The model under review builds one solid part; all positions refer to its coordinate system, in mm. Coordinates: 2 decimals unless noted, no trailing zeros. Order: outer loops, then holes, each group sorted by start corner. A loop starts at its lowest first (then second) coordinate and runs counter-clockwise, first axis right, second up. Notation, with made-up numbers: M 36,56 L 88,56 A20 ccw 88,79 Z; hole C 61,14.25 d4. An arc over 180 degrees is marked long. Answer in a Markdown table with one row per item.
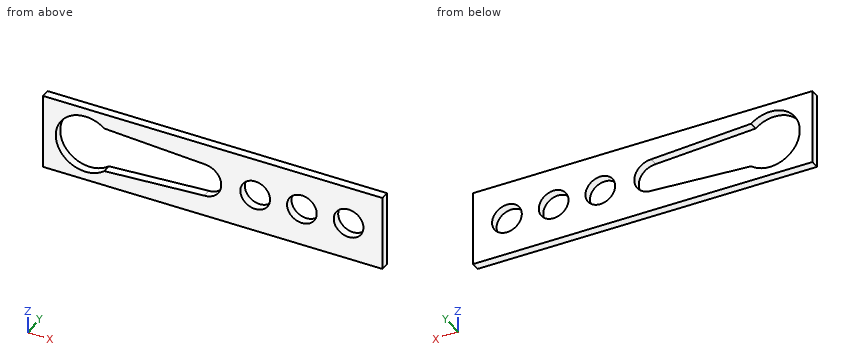
from build123d import *

# Parameters (mm, degrees)
SKETCH2_W           = 40
SKETCH2_H           = 9
BOSS_EXTRUDE1_DEPTH = 1
CUT_EXTRUDE1_DEPTH  = 3
SKETCH4_R           = 1.75
CUT_EXTRUDE2_DEPTH  = 3
LPATTERN1_COUNT     = 3
LPATTERN1_PITCH     = 5.5


with BuildPart() as part:
    # Sketch2 → Boss-Extrude1 (new body)
    with BuildSketch(Plane(origin=(0, 0, 0), x_dir=(1, 0, 0), z_dir=(0, 1, 0))):
        Rectangle(SKETCH2_W, SKETCH2_H)
    extrude(amount=BOSS_EXTRUDE1_DEPTH)

    # Sketch3 → Cut-Extrude1 (cut)
    with BuildSketch(Plane(origin=(0, 1, 0), x_dir=(1, 0, 0), z_dir=(0, 1, 0))):
        with BuildLine():
            Line((-12.772894255, -2.7), (-1, -2))
            ThreePointArc((-1, -2), (1, 0), (-1, 2))
            Line((-1, 2), (-12.772894255, 2.7))
            ThreePointArc((-12.772894255, 2.7), (-18.5, 0), (-12.772894255, -2.7))
        make_face()
    extrude(amount=-CUT_EXTRUDE1_DEPTH, mode=Mode.SUBTRACT)

    # Sketch4 → Cut-Extrude2 (cut)
    with BuildSketch(Plane(origin=(0, 1, 0), x_dir=(1, 0, 0), z_dir=(0, 1, 0))):
        with Locations((5, 0)):
            Circle(SKETCH4_R)
    cut_extrude2 = extrude(amount=-CUT_EXTRUDE2_DEPTH, mode=Mode.SUBTRACT)

    # LPattern1: Cut-Extrude2 ×3
    with Locations(*[(i * LPATTERN1_PITCH, 0, 0) for i in range(1, LPATTERN1_COUNT)]):
        add(cut_extrude2, mode=Mode.SUBTRACT)


solid = part.part
(1) Take a section at A-A (x = -15). Write out the cut boundary in (y, z), then the cut area to 3 significant figures.
Report:
| item | result |
|---|---|
| outline | M 0,-4.5 L 1,-4.5 L 1,-3.5 L 0,-3.5 Z; M 0,3.5 L 1,3.5 L 1,4.5 L 0,4.5 Z |
| area | 2.00 mm^2 |
(2) To check wall thickness, follow line 1 (X direction, y = 0.45, z = 0); line 2 (X direction, y = 0.7, z = -1.5); line 3 (Z direction, x = -15, y = 0.45). State the ranges of each line that lie inside material, in increasing order. Write a range as [from, to].
Report:
| item | result |
|---|---|
| line 1 | [-20, -18.5], [1, 3.25], [6.75, 8.75], [12.25, 14.25], [17.75, 20] |
| line 2 | [-20, -18.16], [0.32, 4.1], [5.9, 9.6], [11.4, 15.1], [16.9, 20] |
| line 3 | [-4.5, -3.5], [3.5, 4.5] |
(3) Take a section at D-D (x = 10.5). Write out the cut boundary in (y, z).
Report:
| item | result |
|---|---|
| outline | M 0,-4.5 L 1,-4.5 L 1,-1.75 L 0,-1.75 Z; M 0,1.75 L 1,1.75 L 1,4.5 L 0,4.5 Z |
(4) Take a section at C-C (z = 0). Write out the cut boundary in (x, y), then the cut area to 3 significant figures.
Report:
| item | result |
|---|---|
| outline | M -20,0 L -18.5,0 L -18.5,1 L -20,1 Z; M 1,0 L 3.25,0 L 3.25,1 L 1,1 Z; M 6.75,0 L 8.75,0 L 8.75,1 L 6.75,1 Z; M 12.25,0 L 14.25,0 L 14.25,1 L 12.25,1 Z; M 17.75,0 L 20,0 L 20,1 L 17.75,1 Z |
| area | 10.0 mm^2 |
(5) Take a section at B-B (y = 0.7). Write out the cut boundary in (x, z).
Report:
| item | result |
|---|---|
| outline | M -20,-4.5 L 20,-4.5 L 20,4.5 L -20,4.5 Z; hole M -12.77,-2.7 L -1,-2 A2 ccw -1,2 L -12.77,2.7 A3.5 ccw long Z; hole C 5,0 d3.5; hole C 10.5,0 d3.5; hole C 16,0 d3.5 |
